from build123d import *

# Parameters (mm, degrees)
SKETCH_1_W          = 100
SKETCH_1_H          = 70
EXTRUDE_1_DEPTH     = 5
SKETCH_2_R          = 3
CUT_EXTRUDE_1_DEPTH = 10


with BuildPart() as part:
    # 草图1 → 凸台-拉伸1 (new, symmetric)
    with BuildSketch(Plane.XY):
        Rectangle(SKETCH_1_W, SKETCH_1_H)
    extrude(amount=EXTRUDE_1_DEPTH, both=True)

    # 草图2 → 切除-拉伸1 (cut)
    with BuildSketch(Plane.XY.offset(5)):
        with Locations((-45, 30)):
            Circle(SKETCH_2_R)
    extrude(amount=-CUT_EXTRUDE_1_DEPTH, mode=Mode.SUBTRACT)


solid = part.part
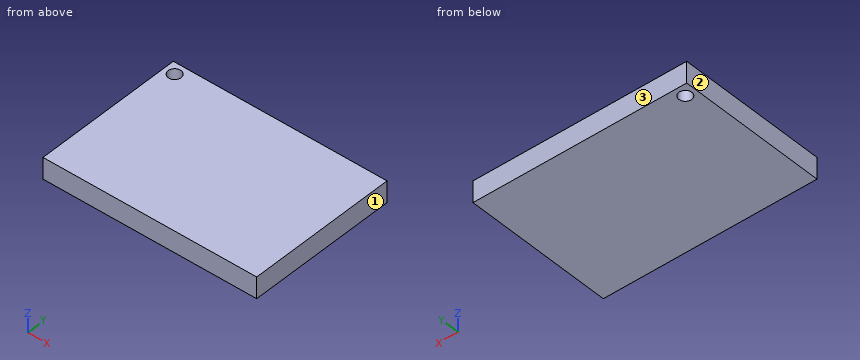
Input: part model. Units: mm. Frame: model coordinates. Face numbers are marked on the shaded views. Round coordinates to 2 decimals unless told otherwise and drop trailing zeros. Order: outer loops, then holes, each group sorted by start corner. A loop starts at its lowest first (then second) coordinate and runs counter-clockwise, first axis right, second up. Notation, with made-up numbers: (11.25, 25.5) - (42.25, 25.5) arc R26 cw to (42.25, 55.5) - close; hole circle Ø4 at (5.25, 1.5). An arc over 180 degrees is marked (long way). Use a Markdown table: item, result.
1. Section B-B on x = -45. Return the cut outline in (y, z).
Evaluation:
| item | result |
|---|---|
| outline | (-35, -5) - (27, -5) - (27, 5) - (-35, 5) - close; (33, -5) - (35, -5) - (35, 5) - (33, 5) - close |
2. Mould query, pull axis X, two halves, no side actions, for the marked faces 1, 2 and 3. Classes: +X half, -X half, draft (parallel to the pull), parting line (faces both ways), or undercut.
Evaluation:
| item | result |
|---|---|
| face 1 | +X half |
| face 2 | -X half |
| face 3 | draft |
3. Material intervals for probe 1 along Y at (x, z) = (-45, -1.5), sorted ascending.
Evaluation:
| item | result |
|---|---|
| probe 1 | -35 to 27, 33 to 35 |
4. Section A-A on y = 30. Return the cut outline in (x, z), then the cut area to 3 significant figures.
Evaluation:
| item | result |
|---|---|
| outline | (-50, -5) - (-48, -5) - (-48, 5) - (-50, 5) - close; (-42, -5) - (50, -5) - (50, 5) - (-42, 5) - close |
| area | 940 mm^2 |
